```python
from build123d import *

# Parameters (mm, degrees)
SKETCH_W         = 30
SKETCH_H         = 50
PAD_DEPTH        = 2.5
SKETCH001_W      = 50
SKETCH001_H      = 25
PAD001_DEPTH     = 2.5
PAD002_DEPTH     = 2
PAD003_DEPTH     = 1
PAD004_DEPTH     = 2
HOLE_D           = 4.4
HOLE_DEPTH       = 25
HOLE_CSINK_D     = 8
HOLE_CSINK_ANGLE = 90


with BuildPart() as part:
    # Sketch → Pad (new body)
    with BuildSketch(Plane.XY):
        with Locations((15, 25)):
            Rectangle(SKETCH_W, SKETCH_H)
    extrude(amount=PAD_DEPTH)

    # Sketch001 → Pad001 (join)
    with BuildSketch(Plane(origin=(0, 0, 0), x_dir=(0, -1, 0), z_dir=(-1, 0, 0))):
        with Locations((-25, 15)):
            Rectangle(SKETCH001_W, SKETCH001_H)
    extrude(amount=-PAD001_DEPTH)

    # Sketch002 → Pad002 (join)
    with BuildSketch(Plane.XZ):
        Polygon((2.5, 2.5), (2.5, 27.5), (30, 2.5), align=None)
    extrude(amount=-PAD002_DEPTH)

    # Sketch003 → Pad003 (join, symmetric)
    with BuildSketch(Plane.XZ.offset(-25)):
        Polygon((2.5, 2.5), (2.5, 27.5), (30, 2.5), align=None)
    extrude(amount=PAD003_DEPTH, both=True)

    # Sketch004 → Pad004 (join)
    with BuildSketch(Plane.XZ.offset(-50)):
        Polygon((2.5, 27.5), (2.5, 2.5), (30, 2.5), align=None)
    extrude(amount=PAD004_DEPTH)

    # Hole
    with Locations(Plane.XY.offset(5)):
        with Locations((16.25, 37), (16.25, 13)):
            CounterSinkHole(HOLE_D / 2, HOLE_CSINK_D / 2, depth=HOLE_DEPTH, counter_sink_angle=HOLE_CSINK_ANGLE)


solid = part.part
```
The listing builds one solid part. Answer for the finished solid, in the listing's coordinates (mm). A direction names the side the tool comes from. Round coordinates to 2 decimals unless told otherwise and drop trailing zeros. Loops run counter-clockwise (first coordinate to the right, second up) from the corner with the lowest first, then second, coordinate; pieces in that order, holes last.
Q1. Find the intervals of material crossed by line 1 (Y direction, x = 15.5, z = 13); line 2 (Y direction, x = 16.25, z = 1.3); line 3 (Z direction, x = 11.25, y = 43), in increasing order.
Q2. Section B-B, the plane y = 37 is taken. Determine the outline of the cut face in (x, z), then the cut area to 4 significant figures.
Q3. Section D-D, the plane x = 4.5 is taken. Determine the outline of the cut face in (y, z).
Q4. Given pin 1 Ø2.5 at (x, y) = (16.25, 13) entering from -Z; pin 2 Ø8 at (x, y) = (16.5, 14.5) entering from +Z; pin 3 Ø1.5 at (x, y) = (10, 25.5) entering from +Z; pin 4 Ø11 at (y, z) = (17.5, 18.5) entering from +X, each flat-ended and moving along its own axis, determine where each tip first touches the part or whether it passes through.
Q5. Section A-A, the plane x = 16.25 is taken. Determine the outline of the cut face in (y, z), then the cut area to 3 significant figures.
Q6. For a pull along X with two mould halves and no side action, classify faces 1 (the face through (30, 25, 1)), 2 (the face through (16.727, 34.852, 1.232)), 3 (the face through (14.15, 13.66, 1.23)), 4 (the face through (10, 26, 10)) as released by +X, released by -X, zero draft, split by the parting line, or undercut.
Q7. Which of the six approach directions +Z, -Z, +X, -X, +Y, -Y give full straight-line access (tool end or side, diameter ignored) to faces 5 (the face through (2.5, 13, 15)), 6 (the face through (15, 25, 0))?
Q8. Section C-C, the plane z = 19 is taken. Determine the outline of the cut face in (x, y), then the cut area to 3 significant figures.
Completed:
1. line 1: y = 0 to 2, 24 to 26, 48 to 50
1. line 2: y = 0 to 10.8, 15.2 to 34.8, 39.2 to 50
1. line 3: z = 0 to 2.5
2. outline: (0, 0) - (14.05, 0) - (14.05, 2.5) - (2.5, 2.5) - (2.5, 27.5) - (0, 27.5) - close; (18.45, 0) - (30, 0) - (30, 2.5) - (18.45, 2.5) - close
2. area: 126.5 mm2
3. outline: (0, 0) - (50, 0) - (50, 25.68) - (48, 25.68) - (48, 2.5) - (26, 2.5) - (26, 25.68) - (24, 25.68) - (24, 2.5) - (2, 2.5) - (2, 25.68) - (0, 25.68) - close
4. pin 1: passes through
4. pin 2: stops at z = 2.5
4. pin 3: stops at z = 21.36
4. pin 4: stops at x = 2.5
5. outline: (0, 0) - (10.8, 0) - (10.8, 2.5) - (2, 2.5) - (2, 15) - (0, 15) - close; (15.2, 0) - (34.8, 0) - (34.8, 2.5) - (26, 2.5) - (26, 15) - (24, 15) - (24, 2.5) - (15.2, 2.5) - close; (39.2, 0) - (50, 0) - (50, 15) - (48, 15) - (48, 2.5) - (39.2, 2.5) - close
5. area: 178 mm2
6. face 1: released by +X
6. face 2: undercut
6. face 3: undercut
6. face 4: zero draft
7. face 5: +Z, +X
7. face 6: -Z, +X, -X, +Y, -Y
8. outline: (0, 0) - (11.85, 0) - (11.85, 2) - (2.5, 2) - (2.5, 24) - (11.85, 24) - (11.85, 26) - (2.5, 26) - (2.5, 48) - (11.85, 48) - (11.85, 50) - (0, 50) - close
8. area: 181 mm2
